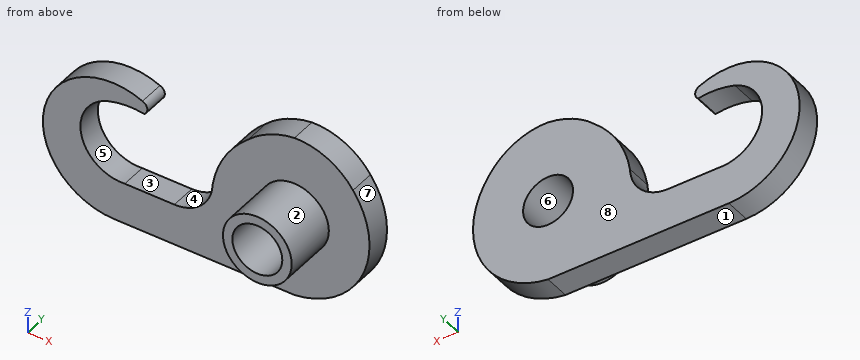
from build123d import *

# Parameters (mm, degrees)
F0_R     = 1.9939
F1_DEPTH = 2.032
F2_R     = 2.7432
F2_R_2   = 1.9939
F3_DEPTH = 4.318


with BuildPart() as f1:
    # F0 (on Front) → F1 (new body)
    with BuildSketch(Plane.XZ):
        with BuildLine():
            ThreePointArc((-3.6886774906, 4.7892003296), (-5.5707472579, 2.5336299725), (-6.5360625118, -0.2408881307))
            ThreePointArc((-6.5360625118, -0.2408881307), (-7.4509999469, -2.3544476099), (-9.5834042014, -3.2245604059))
            Line((-9.5834042014, -3.2245604059), (-13.5428459747, -3.2245604059))
            ThreePointArc((-13.5428459747, -3.2245604059), (-17.0080191324, -0.6859563699), (-14.9047917892, 3.0594902266))
            ThreePointArc((-14.9047917892, 3.0594902266), (-13.4518007595, 3.3451320132), (-11.9730629795, 3.2669735805))
            ThreePointArc((-11.9730629795, 3.2669735805), (-11.746814986, 3.8173410062), (-12.1273721857, 4.2747999394))
            ThreePointArc((-12.1273721857, 4.2747999394), (-19.9550226734, 0.2868008558), (-14.4265317516, -6.5405))
            Line((-14.4265317516, -6.5405), (0, -6.5405))
            ThreePointArc((0, -6.5405), (5.4303827393, -2.4959803043), (4.6703001439, 4.2322788102))
            ThreePointArc((4.6703001439, 4.2322788102), (2.6335498908, 5.9901516108), (0, 6.5405))
            ThreePointArc((0, 6.5405), (-1.9875582205, 5.9665063938), (-3.6886774906, 4.7892003296))
        make_face()
        Circle(F0_R, mode=Mode.SUBTRACT)
    extrude(amount=-F1_DEPTH)

    # F2 (on face) → F3 (join)
    with BuildSketch(Plane.XZ):
        Circle(F2_R)
        Circle(F2_R_2, mode=Mode.SUBTRACT)
    extrude(amount=F3_DEPTH)


solid = f1.part
Input: part model. Units: mm. Frame: model coordinates. Face numbers are marked on the shaded views. A direction names the side the tool comes from. Coordinates: 2 decimals unless noted, no trailing zeros. Loops run counter-clockwise (first coordinate to the right, second up) from the corner with the lowest first, then second, coordinate; pieces in that order, holes last. Notation, with made-up numbers: (63.25, 79.25) - (114.25, 79.25) arc R35 ccw to (114.25, 116.25) - close; hole circle Ø11 at (1, 13.5). An arc over 180 degrees is marked (long way). Answer in a Markdown table with one row per item. Add a question column.
Item 1: Section query A-A on y = 1.75. Return the cut outline in (x, z), then the cut area to 3 significant figures.
Item 2: Mould query, pull axis Z, two halves, no side actions, for the marked faces 5, 6, 7 and 8. Classes: released by +Z, released by -Z, zero draft, split by the parting line, or undercut.
Item 3: Access query for the marked faces 1, 2, 3 and 4. Directions: +Z, -Z, +X, -X, +Y, -Y. A direction counts if a zero-diameter tool reaches every point of the face in a straight line with its end or side. Return the directions, or none.
Item 4: Section query B-B on z = 0. Return the cut outline in (x, y).
Item 5: Line query: line 1 along Z through (x, y) = (0, -0.5); line 2 along Y through (x, z) = (-2, 4.5); line 3 along X through (y, z) = (-3, 0.5). Output: solid intervals per line, ascending. Write a range as [from, to].
Item 6: Section query C-C on x = -15.75. Return the cut outline in (y, z), then the cut area to 3 significant figures.
Item 7: Section query D-D on z = 2.5. Return the cut outline in (x, y).
Item 8: Contact query for flat-ended pins moving along their axis: P1, Ø1.5, axis at y = -0.5, z = 3, coming from the +X side; P2, Ø0.6, axis at x = -12.5, y = 1.5, coming from the +Z side; P3, Ø1.5, axis at x = -4.5, y = -0.5, coming from the +Z side. Output: stop coordinate, or through.
Recorded:
| question | item | result |
|---|---|---|
| 1 | outline | (-14.9, 3.06) arc R6.01 cw to (-11.97, 3.27) arc R0.58 ccw to (-12.13, 4.27) arc R5.65 ccw (long way) to (-14.43, -6.54) - (0, -6.54) arc R6.8 ccw to (4.67, 4.23) arc R5.37 ccw to (0, 6.54) arc R6.41 ccw to (-3.69, 4.79) arc R8.19 ccw to (-6.54, -0.24) arc R3.05 cw to (-9.58, -3.22) - (-13.54, -3.22) arc R3.24 cw to start; hole circle Ø3.99 at (0, 0) |
| 1 | area | 190 mm^2 |
| 2 | face 5 | undercut |
| 2 | face 6 | undercut |
| 2 | face 7 | split by the parting line |
| 2 | face 8 | zero draft |
| 3 | face 1 | -Z, +X, -X, +Y, -Y |
| 3 | face 2 | -Y |
| 3 | face 3 | +Y, -Y |
| 3 | face 4 | +Z, +Y, -Y |
| 4 | outline | (-20.01, 0) - (-17.08, 0) - (-17.08, 2.03) - (-20.01, 2.03) - close; (-6.49, 0) - (-2.74, 0) - (-2.74, -4.32) - (-1.99, -4.32) - (-1.99, 2.03) - (-6.49, 2.03) - close; (1.99, -4.32) - (2.74, -4.32) - (2.74, 0) - (5.99, 0) - (5.99, 2.03) - (1.99, 2.03) - close |
| 5 | line 1 | [-2.74, -1.99], [1.99, 2.74] |
| 5 | line 2 | [0, 2.03] |
| 5 | line 3 | [-2.7, -1.93], [1.93, 2.7] |
| 6 | outline | (0, -6.38) - (2.03, -6.38) - (2.03, -2.62) - (0, -2.62) - close; (0, 2.62) - (2.03, 2.62) - (2.03, 4.61) - (0, 4.61) - close |
| 6 | area | 11.7 mm^2 |
| 7 | outline | (-18.95, 0) - (-15.9, 0) - (-15.9, 2.03) - (-18.95, 2.03) - close; (-5.59, 0) - (-1.13, 0) - (-1.13, -4.32) - (1.13, -4.32) - (1.13, 0) - (5.59, 0) - (5.59, 2.03) - (-5.59, 2.03) - close |
| 8 | P1 | x = 5.61 |
| 8 | P2 | z = 4.52 |
| 8 | P3 | z = 4.57 |
